Check sheet for the modelled part. Datum: model origin and axes. Units: mm. A direction names the side the tool comes from. Give positions to 0.01 mm unless a question says otherwise; leave off trailing zeros. Order: outer loops, then holes, each group sorted by start corner. A loop starts at its lowest first (then second) coordinate and runs counter-clockwise, first axis right, second up. Notation, with made-up numbers: (18, 59.25) -> (50, 59.25) arc R16 ccw to (50, 85.25) -> close; hole circle Ø4 at (-8, 10.5). An arc over 180 degrees is marked (long way). Answer in a Markdown table with one row per item. Add a question column.
(1) Cross-section at A-A (z = -26). Record the cut outline in (x, y), then the cut area to 3 significant figures.
(2) Cross-section at B-B (x = -60.5). Record the cut outline in (y, z), then the cut area to 3 significant figures.
(3) Thickness scan on L1, parallel to Z at x = 87.4, y = 1.3; L2, parallel to X at y = 2.05, z = 50.9; L3, parallel to Z at x = -87.4, y = 3.1. Record the ranges inside material, lowest first. Write a range as [from, to].
(4) Cross-section at D-D (z = -1.5). Record the cut outline in (x, y).
(5) Release check for a two-part mould opening along Z. For faces 1 (the face through (-40.8, 2, -33)), 2 (the face through (-87, -9.6, -33)), 3 (the face through (-48, 1.5, -33)), 4 (the face through (92.719, 2.028, 55.594)) record: released by +Z, released by -Z, zero draft, split by the parting line, or undercut.
(6) Go/stop test with flat-tipped pins: pin 1 (1.2 mm diameter, centred on y = -1, z = -37, fed in from -X); pin 2 (6 mm diameter, centred on x = -58, y = -7.5, fed in from -Z); pin 3 (7.5 mm diameter, centred on x = -91.5, y = -1.5, fed in from -Z); pin 4 (1.3 mm diameter, centred on y = -5, z = -19.5, fed in from +X). Record where each tip stops, or that it passes through.
(7) Set-up check for faces 5 (the face through (-65, -2, -14.75)), 6 (the face through (-67, 2, -18.7)), 7 (the face through (-87, -5, -47.8)): record each of +Z, -Z, +X, -X, +Y, -Y from which the full face is reachable in a straight line by a thin tool's end or side.
(8) Cross-section at C-C (x = -26). Record the cut outline in (y, z).
```python
from build123d import *

# Parameters (mm, degrees)
SKETCH_1_W          = 272.533053494
SKETCH_1_H          = 136.587531522
EXTRUDE_1_DEPTH     = 4
SKETCH_2_W          = 272.533053494
SKETCH_2_H          = 136.587531522
CUT_EXTRUDE_1_DEPTH = 4
CUT_EXTRUDE_2_DEPTH = 4
CUT_EXTRUDE_3_DEPTH = 4
SKETCH_5_W          = 34
SKETCH_5_H          = 36
EXTRUDE_2_DEPTH     = 4
SKETCH_6_W          = 13.2
SKETCH_6_H          = 4
EXTRUDE_3_DEPTH     = 5.6
SKETCH_7_W          = 17.2
SKETCH_7_H          = 30.1
EXTRUDE_4_DEPTH     = 4
SKETCH_8_W          = 5
SKETCH_8_H          = 27.5
CUT_EXTRUDE_4_DEPTH = 4
SKETCH_9_W          = 27.5
SKETCH_9_H          = 2.5
CUT_EXTRUDE_5_DEPTH = 4
SKETCH_10_R         = 1.6
CUT_EXTRUDE_6_DEPTH = 10
SKETCH_13_W         = 15
SKETCH_13_H         = 15
CUT_EXTRUDE_7_DEPTH = 5


with BuildPart() as part:
    # 草图1 → 凸台-拉伸1 (new body)
    with BuildSketch(Plane(origin=(0, 0, 0), x_dir=(1, 0, 0), z_dir=(0, 1, 0))):
        Rectangle(SKETCH_1_W, SKETCH_1_H)
    extrude(amount=EXTRUDE_1_DEPTH)

    # 草图2 → 切除-拉伸1 (cut)
    with BuildSketch(Plane(origin=(0, 4, 0), x_dir=(1, 0, 0), z_dir=(0, 1, 0))):
        Rectangle(SKETCH_2_W, SKETCH_2_H)
        with BuildLine():
            Line((-87, 58), (87, 58))
            ThreePointArc((87, 58), (92.656854249, 55.656854249), (95, 50))
            Line((95, 50), (95, -50))
            ThreePointArc((95, -50), (92.656854249, -55.656854249), (87, -58))
            Line((87, -58), (-87, -58))
            ThreePointArc((-87, -58), (-92.656854249, -55.656854249), (-95, -50))
            Line((-95, -50), (-95, 50))
            ThreePointArc((-95, 50), (-92.656854249, 55.656854249), (-87, 58))
        make_face(mode=Mode.SUBTRACT)
    extrude(amount=-CUT_EXTRUDE_1_DEPTH, mode=Mode.SUBTRACT)

    # 草图3 → 切除-拉伸2 (cut)
    with BuildSketch(Plane.XZ):
        Polygon((-95, -22), (-81.8, -22), (-81.8, -19), (-51.8, -19), (-51.8, -46.5), (-81.8, -46.5), (-81.8, -43.5), (-95, -43.5), align=None)
    extrude(amount=-CUT_EXTRUDE_2_DEPTH, mode=Mode.SUBTRACT)

    # 草图4 → 切除-拉伸3 (cut)
    with BuildSketch(Plane.XZ):
        Polygon((-51.5, -18.7), (-51.5, -46.8), (-82.1, -46.8), (-82.1, -43.8), (-95, -43.8), (-95, -21.7), (-82.1, -21.7), (-82.1, -18.7), align=None)
    extrude(amount=-CUT_EXTRUDE_3_DEPTH, mode=Mode.SUBTRACT)

    # 草图5 → 凸台-拉伸2 (add)
    with BuildSketch(Plane.XZ):
        with Locations((-64.8, -32.75)):
            Rectangle(SKETCH_5_W, SKETCH_5_H)
    extrude(amount=EXTRUDE_2_DEPTH)

    # 草图6 → 凸台-拉伸3 (add)
    with BuildSketch(Plane.XZ):
        with Locations((-88.4, -19.7)):
            Rectangle(SKETCH_6_W, SKETCH_6_H)
        with Locations((-88.4, -45.8)):
            Rectangle(SKETCH_6_W, SKETCH_6_H)
    extrude(amount=EXTRUDE_3_DEPTH)

    # 草图7 → 凸台-拉伸4 (add)
    with BuildSketch(Plane.XZ.offset(5.6)):
        with Locations((-86.4, -32.75)):
            Rectangle(SKETCH_7_W, SKETCH_7_H)
    extrude(amount=EXTRUDE_4_DEPTH)

    # 草图8 → 切除-拉伸4 (cut)
    with BuildSketch(Plane(origin=(0, 4, 0), x_dir=(1, 0, 0), z_dir=(0, 1, 0))):
        with Locations((-43.3, 32.75)):
            Rectangle(SKETCH_8_W, SKETCH_8_H)
    extrude(amount=-CUT_EXTRUDE_4_DEPTH, mode=Mode.SUBTRACT)

    # 草图9 → 切除-拉伸5 (cut)
    with BuildSketch(Plane(origin=(-45.8, 0, 0), x_dir=(0, 0, -1), z_dir=(1, 0, 0))):
        with Locations((32.75, 2.75)):
            Rectangle(SKETCH_9_W, SKETCH_9_H)
    extrude(amount=-CUT_EXTRUDE_5_DEPTH, mode=Mode.SUBTRACT)

    # 草图10 → 切除-拉伸6 (cut)
    with BuildSketch(Plane(origin=(0, 4, 0), x_dir=(1, 0, 0), z_dir=(0, 1, 0))):
        with Locations(Location((87.4, 50.9, 0), (0, 0, 270))):
            Circle(SKETCH_10_R)
        with Locations(Location((-87.4, 50.9, 0), (0, 0, 270))):
            Circle(SKETCH_10_R)
        with Locations(Location((-87.4, -50.9, 0), (0, 0, 270))):
            Circle(SKETCH_10_R)
        with Locations(Location((87.4, -50.9, 0), (0, 0, 270))):
            Circle(SKETCH_10_R)
    extrude(amount=-CUT_EXTRUDE_6_DEPTH, mode=Mode.SUBTRACT)

    # 草图13 → 切除-拉伸7 (cut, symmetric)
    with BuildSketch(Plane.XZ):
        with Locations((72.5, 50.5)):
            Rectangle(SKETCH_13_W, SKETCH_13_H)
        with Locations((-72.5, 50.5)):
            Rectangle(SKETCH_13_W, SKETCH_13_H)
    extrude(amount=CUT_EXTRUDE_7_DEPTH, both=True, mode=Mode.SUBTRACT)


solid = part.part
```
Answer below:
| question | item | result |
|---|---|---|
| 1 | outline | (-95, -9.6) -> (-77.8, -9.6) -> (-77.8, -5.6) -> (-95, -5.6) -> close; (-81.8, -4) -> (-47.8, -4) -> (-47.8, 0) -> (-45.8, 0) -> (-45.8, 1.5) -> (-49.8, 1.5) -> (-49.8, 4) -> (-51.5, 4) -> (-51.5, 0) -> (-81.8, 0) -> close; (-40.8, 0) -> (95, 0) -> (95, 4) -> (-40.8, 4) -> close |
| 1 | area | 761 mm² |
| 2 | outline | (-4, -50.75) -> (0, -50.75) -> (0, -58) -> (4, -58) -> (4, -46.8) -> (0, -46.8) -> (0, -18.7) -> (4, -18.7) -> (4, 58) -> (0, 58) -> (0, -14.75) -> (-4, -14.75) -> close |
| 2 | area | 496 mm² |
| 3 | L1 | z = [-57.99, -52.5], [-49.3, 49.3], [52.5, 57.99] |
| 3 | L2 | x = [-94.95, -89], [-85.8, -80], [-65, 65], [80, 85.8], [89, 94.95] |
| 3 | L3 | z = [-57.99, -52.5], [-49.3, -43.8], [-21.7, 49.3], [52.5, 57.99] |
| 4 | outline | (-95, 0) -> (95, 0) -> (95, 4) -> (-95, 4) -> close |
| 5 | face 1 | undercut |
| 5 | face 2 | zero draft |
| 5 | face 3 | undercut |
| 5 | face 4 | released by +Z |
| 6 | pin 1 | stops at x = -81.8 |
| 6 | pin 2 | passes through |
| 6 | pin 3 | stops at z = -57.93 |
| 6 | pin 4 | stops at x = -77.8 |
| 7 | face 5 | +Z, +X, -X, -Y |
| 7 | face 6 | +Y |
| 7 | face 7 | -Z, -X, -Y |
| 8 | outline | (0, -58) -> (4, -58) -> (4, 58) -> (0, 58) -> close |
